Input: part model. Units: mm. Frame: model coordinates. A direction names the side the tool comes from. Give positions to 0.01 mm unless a question says otherwise; leave off trailing zeros. Loops run counter-clockwise (first coordinate to the right, second up) from the corner with the lowest first, then second, coordinate; pieces in that order, holes last. Notation, with made-up numbers: (16.25, 42) -> (61.25, 42) arc R28 cw to (61.25, 76) -> close; hole circle Ø5 at (32.5, -19). An arc over 180 degrees is marked (long way). Answer as a JSON object with one key per item and string values.
```python
from build123d import *

# Parameters (mm, degrees)
F0_W     = 523.5
F0_H     = 72
F1_DEPTH = 43
F2_W     = 93
F2_H     = 25
F3_DEPTH = 93
F4_W     = 523.5
F4_H     = 14
F5_DEPTH = 17.5


with BuildPart() as f1:
    # F0 (on Front) → F1 (new body)
    with BuildSketch(Plane.XZ):
        Rectangle(F0_W, F0_H)
    extrude(amount=F1_DEPTH)

    # F2 (on face) → F3 (cut)
    with BuildSketch(Plane.XZ.offset(43)):
        with Locations((-215.25, -23.5)):
            Rectangle(F2_W, F2_H)
        with Locations((215.25, -23.5)):
            Rectangle(F2_W, F2_H)
    extrude(amount=-F3_DEPTH, mode=Mode.SUBTRACT)

    # F4 (on face) → F5 (join)
    with BuildSketch(Plane(origin=(0, 0, 0), x_dir=(-1, 0, 0), z_dir=(0, 1, 0))):
        with Locations((0, 29)):
            Rectangle(F4_W, F4_H)
    extrude(amount=F5_DEPTH)


solid = f1.part
```
Q1. Pin query (flat end, axial travel): pin 1 (14 mm diameter, centred on x = -128.5, y = 9, fed in from -Z); pin 2 (21.5 mm diameter, centred on x = -196, y = -11.5, fed in from -Z); pin 3 (7.5 mm diameter, centred on y = -12.5, z = -18.5, fed in from -X). Return the tip coordinate at first contact, or that it passes through.
Evaluation:
{"pin 1": "stops at z = 22", "pin 2": "stops at z = -11", "pin 3": "stops at x = -168.75"}
Q2. Section A-A, the plane y = -11. Return the cut outline in (x, z).
Evaluation:
{"outline": "(-261.75, -11) -> (-168.75, -11) -> (-168.75, -36) -> (168.75, -36) -> (168.75, -11) -> (261.75, -11) -> (261.75, 36) -> (-261.75, 36) -> close"}
Q3. Section D-D, the plane z = -20. Return the cut outline in (x, y).
Evaluation:
{"outline": "(-168.75, -43) -> (168.75, -43) -> (168.75, 0) -> (-168.75, 0) -> close"}
Q4. Ray query, line 1 along Y through (x, z) = (-86.5, -31); line 2 along X through (y, z) = (-17, -31.5); line 3 along Z through (x, y) = (-172.5, -3.5). Return the intervals inside material, ascending.
Evaluation:
{"line 1": "y = -43 to 0", "line 2": "x = -168.75 to 168.75", "line 3": "z = -11 to 36"}
Q5. Section C-C, the plane z = 16.5. Return the cut outline in (x, y), then the cut area to 3 significant figures.
Evaluation:
{"outline": "(-261.75, -43) -> (261.75, -43) -> (261.75, 0) -> (-261.75, 0) -> close", "area": "22,500 mm2"}
Q6. Section B-B, the plane x = 183. Return the cut outline in (y, z).
Evaluation:
{"outline": "(-43, -11) -> (0, -11) -> (0, 22) -> (17.5, 22) -> (17.5, 36) -> (-43, 36) -> close"}
Q7. Access query for faces 1 (the flat face through (168.75, -22, -24)), 2 (the flat face through (261.75, -20, 12)), 3 (the flat face through (-168.75, -22, -24)), 4 (the flat face through (-4, -43, 9)), 5 (the flat face through (-4, 0, 0)). Directions: +Z, -Z, +X, -X, +Y, -Y. A direction counts if a zero-diameter tool reaches every point of the face in a straight line with its end or side. Return the directions, or none.
Evaluation:
{"face 1": "-Z, +X, +Y, -Y", "face 2": "+Z, -Z, +X, +Y, -Y", "face 3": "-Z, -X, +Y, -Y", "face 4": "+Z, -Z, +X, -X, -Y", "face 5": "-Z, +X, -X, +Y"}
